```python
from build123d import *

# Parameters (mm, degrees)
SKETCH_1_W          = 200
SKETCH_1_H          = 60
EXTRUDE_1_DEPTH     = 2
SKETCH_3_R          = 2.55
CUT_EXTRUDE_1_DEPTH = 105.422219858
CUT_EXTRUDE_2_DEPTH = 96.828733232
SKETCH_5_R          = 17.5
CUT_EXTRUDE_3_DEPTH = 0.2
FILLET_1_R          = 3


with BuildPart() as part:
    # 草图1 → 凸台-拉伸1 (new body)
    with BuildSketch(Plane(origin=(0, 0, 0), x_dir=(1, 0, 0), z_dir=(0, 1, 0))):
        Rectangle(SKETCH_1_W, SKETCH_1_H)
    extrude(amount=EXTRUDE_1_DEPTH)

    # 草图3 → 切除-拉伸1 (cut, through all)
    with BuildSketch(Plane(origin=(0, 2, 0), x_dir=(1, 0, 0), z_dir=(0, 1, 0))):
        Polygon((82.173464202, -20.771330594), (-77.826535798, -20.771330594), (-86.642884834, 30), (-100, 30), (-100, -30), (100, -30), (100, 30), (90.989813237, 30), align=None)
        with Locations(Location((-74.153372817, 24, 0), (0, 0, 270))):
            Circle(SKETCH_3_R)
        with Locations(Location((-70.731615422, 4.294884514, 0), (0, 0, 270))):
            Circle(SKETCH_3_R)
        with Locations(Location((-67.309858027, -15.410230973, 0), (0, 0, 270))):
            Circle(SKETCH_3_R)
        with Locations(Location((78.50030122, 24, 0), (0, 0, 270))):
            Circle(SKETCH_3_R)
        with Locations(Location((71.65678643, -15.410230973, 0), (0, 0, 270))):
            Circle(SKETCH_3_R)
        with Locations(Location((75.078543825, 4.294884514, 0), (0, 0, 270))):
            Circle(SKETCH_3_R)
    extrude(amount=-CUT_EXTRUDE_1_DEPTH, mode=Mode.SUBTRACT)

    # 草图4 → 切除-拉伸2 (cut, through all)
    with BuildSketch(Plane.XZ):
        Polygon((76.083674975, 20.771330594), (84.90002401, -30), (90.989813237, -30), (82.173464202, 20.771330594), align=None)
        Polygon((-86.642884834, -30), (-80.553095607, -30), (-71.736746572, 20.771330594), (-77.826535798, 20.771330594), align=None)
    extrude(amount=-CUT_EXTRUDE_2_DEPTH, mode=Mode.SUBTRACT)

    # 草图5 → 切除-拉伸3 (cut)
    with BuildSketch(Plane.XZ):
        with Locations(Location((-6, -3, 0), (0, 0, 270))):
            Circle(SKETCH_5_R)
    extrude(amount=-CUT_EXTRUDE_3_DEPTH, mode=Mode.SUBTRACT)

    # 圆角1
    fillet_1_edges = [part.edges().sort_by_distance(p)[0] for p in [
        (-80.553095607, 1, -30),
        (-71.736746572, 1, 20.771330594),
        (84.90002401, 1, -30),
        (76.083674975, 1, 20.771330594),
    ]]
    fillet(fillet_1_edges, radius=FILLET_1_R)


solid = part.part
```
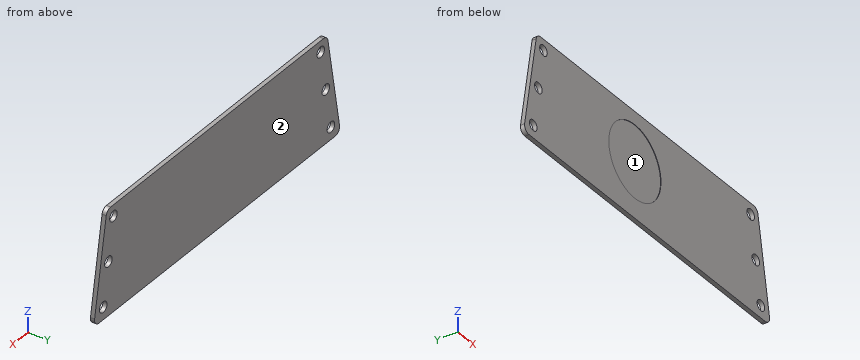
Geometry: final body of the model. Coordinates: model frame, mm. Face numbers are marked on the shaded views. Round coordinates to 2 decimals unless told otherwise and drop trailing zeros. Order: outer loops, then holes, each group sorted by start corner. A loop starts at its lowest first (then second) coordinate and runs counter-clockwise, first axis right, second up. Notation, with made-up numbers: (51.5, 72.5) - (58.5, 72.5) arc R26 cw to (58.5, 102.5) - close; hole circle Ø10 at (-36.5, 68.5). An arc over 180 degrees is marked (long way). Write item = value, one per line. Start each with the question number.
Q1. Pin query (flat end, axial travel): pin 1 (2 mm diameter, centred on x = -42.5, z = -13, fed in from -Y); pin 2 (17.5 mm diameter, centred on x = 1, z = -8, fed in from -Y). Return the tip coordinate at first contact, or that it passes through.
Q2. Cut plane D-D on z = -14. Return the cut outline in (x, y).
Q3. Pull-direction query (Z, two-part tool) for the marked faces 1 and 2; classes: +Z half, -Z half, draft (parallel to the pull), parting line (faces both ways), or undercut.
Q4. Cut plane C-C on x = -6. Return the cut outline in (y, z), and give its area (3 significant figures).
Q5. Ray query, line 1 (X direction, y = 1.45, z = -26); line 2 (X direction, y = 0.6, z = 15); line 3 (Y direction, x = -3, z = -6). Return the intervals inside material, ascending. Write a range as from..to.
Q6. Cut plane B-B on z = -24. Return the cut outline in (x, y).
Q7. Cut plane A-A on y = 1.25. Return the cut outline in (x, z).
Outcome:
q1.pin_1 = 0
q1.pin_2 = 0.2
q2.outline = (-77.77, 0) - (-19.61, 0) - (-19.61, 0.2) - (7.61, 0.2) - (7.61, 0) - (82.12, 0) - (82.12, 2) - (-77.77, 2) - close
q3.face_1 = undercut
q3.face_2 = draft
q4.outline = (0, -30) - (2, -30) - (2, 20.77) - (0, 20.77) - (0, 14.5) - (0.2, 14.5) - (0.2, -20.5) - (0, -20.5) - close
q4.area = 94.5 mm^2
q5.line_1 = -79.86..-75.74, -72.57..76.92, 80.08..84.21
q5.line_2 = -72.74..-69.83, -64.79..69.14, 74.17..77.09
q5.line_3 = 0.2..2
q6.outline = (-79.51, 0) - (-76.7, 0) - (-76.7, 2) - (-79.51, 2) - close; (-71.6, 0) - (75.95, 0) - (75.95, 2) - (-71.6, 2) - close; (81.05, 0) - (83.86, 0) - (83.86, 2) - (81.05, 2) - close
q7.outline = (-79.94, -26.49) arc R3 ccw to (-76.99, -30) - (81.33, -30) arc R3 ccw to (84.29, -26.49) - (76.52, 18.28) arc R3 ccw to (73.56, 20.77) - (-69.21, 20.77) arc R3 ccw to (-72.17, 18.28) - close; hole circle Ø5.1 at (-74.15, -24); hole circle Ø5.1 at (-70.73, -4.29); hole circle Ø5.1 at (-67.31, 15.41); hole circle Ø5.1 at (71.66, 15.41); hole circle Ø5.1 at (75.08, -4.29); hole circle Ø5.1 at (78.5, -24)
